Read the model definition and answer for the solid it produces. Units are mm, in the model's axes. Coordinates: 2 decimals unless noted, no trailing zeros. Order: outer loops, then holes, each group sorted by start corner. A loop starts at its lowest first (then second) coordinate and runs counter-clockwise, first axis right, second up. Notation, with made-up numbers: (71.5, -2) - (113.5, -2) arc R15 ccw to (113.5, 2) - close; hole circle Ø1 at (23, 85.25). An arc over 180 degrees is marked (long way). Use one line per item in the form item = value.
```python
from build123d import *

# Parameters (mm, degrees)
F0_R     = 15
F0_R_2   = 55
F1_DEPTH = 25
F2_R     = 55
F3_DEPTH = 5
F4_R     = 6
F5_DEPTH = 25


with BuildPart() as f1:
    # F0 (on Front) → F1 (new body)
    with BuildSketch(Plane.XZ):
        with BuildLine():
            ThreePointArc((78.619082, -14.8), (0, 80), (-78.619082, -14.8))
            Line((-78.619082, -14.8), (-42.257756, -207.955))
            ThreePointArc((-42.257756, -207.955), (0, -243), (42.257756, -207.955))
            Line((42.257756, -207.955), (78.619082, -14.8))
        make_face()
        with Locations((0, -200)):
            Circle(F0_R, mode=Mode.SUBTRACT)
        Circle(F0_R_2, mode=Mode.SUBTRACT)
    extrude(amount=F1_DEPTH)

    # F2 (on face) → F3 (cut)
    with BuildSketch(Plane(origin=(0, 0, 0), x_dir=(-1, 0, 0), z_dir=(0, 1, 0))):
        with BuildLine():
            Line((-78.619082, -14.8), (-64.462722, -90))
            Line((-64.462722, -90), (64.462722, -90))
            Line((64.462722, -90), (78.619082, -14.8))
            ThreePointArc((78.619082, -14.8), (0, 80), (-78.619082, -14.8))
        make_face()
        Circle(F2_R, mode=Mode.SUBTRACT)
    extrude(amount=-F3_DEPTH, mode=Mode.SUBTRACT)

    # F4 (on face) → F5 (cut)
    with BuildSketch(Plane.XZ.offset(25)):
        with Locations((0, 64)):
            Circle(F4_R)
        with Locations((45.254834, 45.254834)):
            Circle(F4_R)
        with Locations((64, 0)):
            Circle(F4_R)
        with Locations((45.254834, -45.254834)):
            Circle(F4_R)
        with Locations((0, -64)):
            Circle(F4_R)
        with Locations((-45.254834, -45.254834)):
            Circle(F4_R)
        with Locations((-64, 0)):
            Circle(F4_R)
        with Locations((-45.254834, 45.254834)):
            Circle(F4_R)
    extrude(amount=-F5_DEPTH, mode=Mode.SUBTRACT)


solid = f1.part
```
(1) The mould has two halves that part along Z. Classify faces 1 (the flat face through (37, -5, -42)), 2 (the cylindrical face through (-0.83, -12.32, -242.99)), 3 (the cylindrical face through (48.48, -15.14, -40.196)), 4 (the cylindrical face through (50.8, -15.14, 42.96)): +Z half, -Z half, draft (parallel to the pull), parting line (faces both ways), or undercut.
Answer list:
face_1 = draft
face_2 = -Z half
face_3 = undercut
face_4 = undercut
(2) Section D-D, the plane y = -8 is taken. State how many separate pieces and enclosed holes the cut face has, then the cut area to 3 significant figures.
Answer list:
separate_pieces = 1
enclosed_holes = 10
area = 26,900 mm2
(3) Given pin 1 Ø6 at (y, z) = (-15.5, 43) entering from -X; pin 2 Ø1 at (y, z) = (-20, -210) entering from -X; pin 3 Ø14 at (x, z) = (45.25, 45.25) entering from +Y; pin 4 Ø8 at (x, z) = (-41.5, -166.5) entering from +Y, each flat-ended and moving along its own axis, determine where each tip first touches the part or whether it passes through.
Answer list:
pin_1 = -69.28
pin_2 = -41.94
pin_3 = -5
pin_4 = 0
(4) Section A-A, the plane z = 0 is taken. Write down the section's boundary in (x, y).
Answer list:
outline = (-80, -25) - (-70, -25) - (-70, -5) - (-80, -5) - close; (-58, -25) - (-55, -25) - (-55, -5) - (-58, -5) - close; (55, -25) - (58, -25) - (58, -5) - (55, -5) - close; (70, -25) - (80, -25) - (80, -5) - (70, -5) - close
(5) Section C-C, the plane z = 64 is taken. Write down the section's boundary in (x, y).
Answer list:
outline = (-48, -25) - (-6, -25) - (-6, -5) - (-48, -5) - close; (6, -25) - (48, -25) - (48, -5) - (6, -5) - close
(6) Section B-B, the plane x = 0 is taken. Write down the section's boundary in (y, z), then the cut area to 4 significant figures.
Answer list:
outline = (-25, -243) - (0, -243) - (0, -215) - (-25, -215) - close; (-25, -185) - (0, -185) - (0, -90) - (-5, -90) - (-5, -70) - (-25, -70) - close; (-25, -58) - (-5, -58) - (-5, -55) - (-25, -55) - close; (-25, 55) - (-5, 55) - (-5, 58) - (-25, 58) - close; (-25, 70) - (-5, 70) - (-5, 80) - (-25, 80) - close
area = 3,795 mm2
(7) Straight lines are drawn through the part: L1, parallel to Z at x = 0, y = -20; L2, parallel to X at y = -7.5, z = -49.5; L3, parallel to Z at x = 5, y = -7. For each, find the intervals that lie inside material, in ascending order.
Answer list:
L1 = -243 to -215, -185 to -70, -58 to -55, 55 to 58, 70 to 80
L2 = -72.09 to -49.49, -41.01 to -23.97, 23.97 to 41.01, 49.49 to 72.09
L3 = -242.71 to -214.14, -185.86 to -67.32, -60.68 to -54.77, 54.77 to 60.68, 67.32 to 79.84
